Part print with two shaded views. Sizes in mm from the minimum x, y, z corner. Round coordinates to 2 decimals unless told otherwise and drop trailing zeros. Write each loop counter-clockwise with the first axis right and the second up, starting at its lowest first coordinate (ties: lowest second). Pieces come first, ordered by that corner, then holes. Notation, with made-up numbers: (-20, 20.25) -> (22, 20.25) arc R28 ccw to (22, 54.25) -> close; hole circle Ø7 at (-22.5, 12.5). An arc over 180 degrees is marked (long way). Return JSON: item names as keys, results as strings.
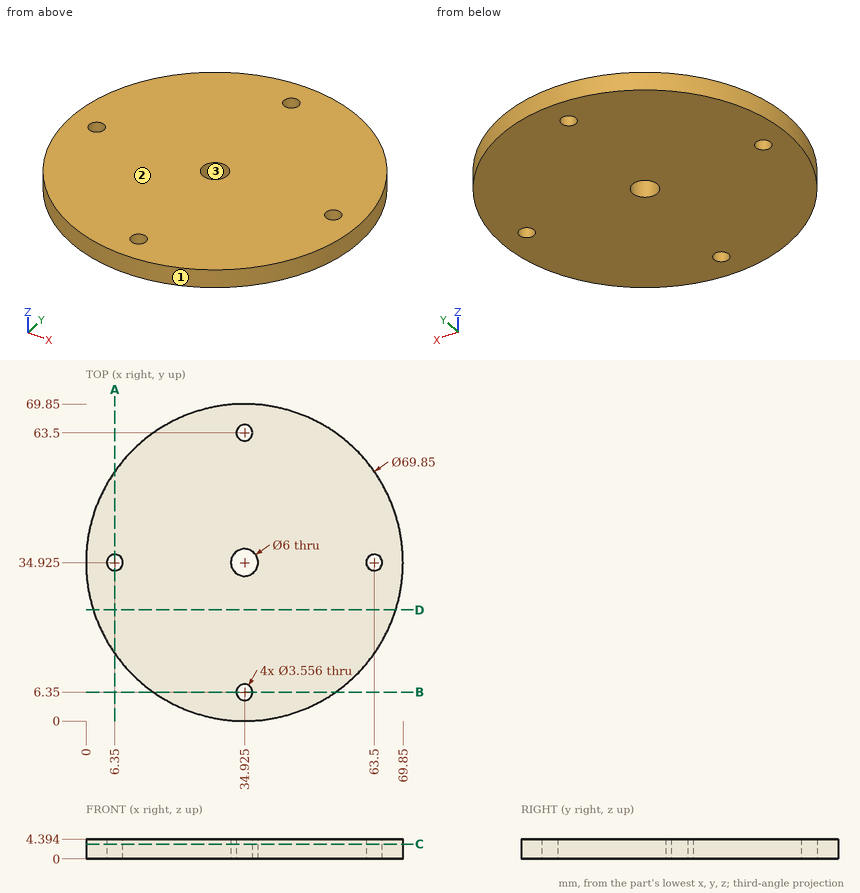
Q1. Wall check: L1, parallel to X at y = 33.5, z = 1.7 (1 decimal); L2, parallel to Y at x = 6.35, z = 0.95 (1 decimal); L3, parallel to X at y = 23.5, z = 4. Give the ranges that are in metal, low to high.
Verdict:
{"L1": "x = 0 to 5.3, 7.4 to 32.3, 37.6 to 62.4, 64.6 to 69.8", "L2": "y = 14.8 to 33.1, 36.7 to 55", "L3": "x = 1.92 to 67.93"}
Q2. Saw through at D-D on y = 24.5. List the corners of the cut face in (x, z).
Verdict:
{"outline": "(1.59, 0) -> (68.26, 0) -> (68.26, 4.39) -> (1.59, 4.39) -> close"}
Q3. Two-plate mould, pull along X, no slides. Class the marked faces 1, 2 and 3: +X half, -X half, draft (parallel to the pull), parting line (faces both ways), or undercut.
Verdict:
{"face 1": "parting line", "face 2": "draft", "face 3": "undercut"}
Q4. Saw through at C-C on z = 3.25. List the corners of the cut face in (x, y) (3 decimals), then the cut area to 3 significant figures.
Verdict:
{"outline": "circle Ø69.85 at (34.925, 34.925); hole circle Ø3.556 at (6.35, 34.925); hole circle Ø6 at (34.925, 34.925); hole circle Ø3.556 at (34.925, 6.35); hole circle Ø3.556 at (34.925, 63.5); hole circle Ø3.556 at (63.5, 34.925)", "area": "3,760 mm²"}
Q5. Pin check, flat tip, straight feed: pin 1 Ø1 at (y, z) = (23, 2) entering from +X. Stop position of the tip, or through.
Verdict:
{"pin 1": "stops at x = 67.93"}
Q6. Saw through at A-A on x = 6.35. List the corners of the cut face in (y, z), then the cut area to 3 significant figures.
Verdict:
{"outline": "(14.84, 0) -> (33.15, 0) -> (33.15, 4.39) -> (14.84, 4.39) -> close; (36.7, 0) -> (55.01, 0) -> (55.01, 4.39) -> (36.7, 4.39) -> close", "area": "161 mm²"}
